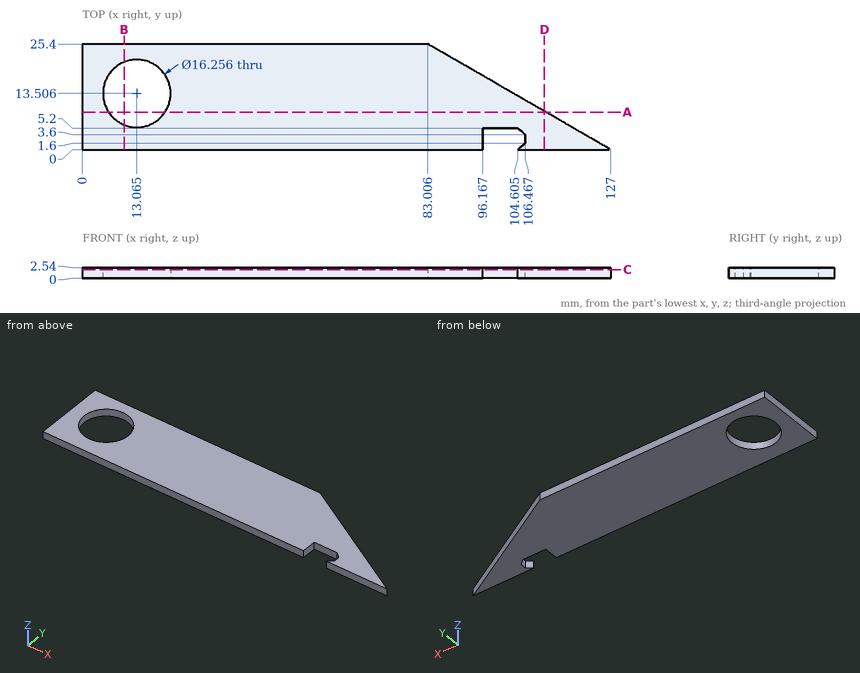
The figure shows three views and two pictorial views of one solid part (mm, origin at its lowest corner). Answer the questions. Give positions to 0.01 mm unless a question says otherwise; leave off trailing zeros. Order: outer loops, then holes, each group sorted by start corner. A loop starts at its lowest first (then second) coordinate and runs counter-clockwise, first axis right, second up. Notation, with made-up numbers: (-39.5, 39) -> (-16.5, 39) arc R28 cw to (-16.5, 59) -> close; hole circle Ø11 at (65.25, -8). An arc over 180 degrees is marked (long way). One line per item, written item: value.
1) Find section C-C, the plane z = 2.05. Determine the outline of the cut face in (x, y) (1 decimal).
Reported:
outline: (0, 0) -> (96.2, 0) -> (96.2, 5.2) -> (104.6, 5.2) -> (106.5, 3.6) -> (106.5, 1.6) -> (104.6, 0) -> (127, 0) -> (83, 25.4) -> (0, 25.4) -> close; hole circle Ø16.3 at (13.1, 13.5)
2) A flat-ended cylindrical pin translates along its axis: P1, Ø12, axis at x = 82, y = 23, coming from the -Z side. Find the tip coordinate at first contact, or state that the pin passes through.
Reported:
P1: stops at z = 0
3) Find section B-B, the plane x = 10. Determine the outline of the cut face in (y, z).
Reported:
outline: (0, 0) -> (5.98, 0) -> (5.98, 2.54) -> (0, 2.54) -> close; (21.03, 0) -> (25.4, 0) -> (25.4, 2.54) -> (21.03, 2.54) -> close
4) Find section D-D, the plane x = 111. Determine the outline of the cut face in (y, z).
Reported:
outline: (0, 0) -> (9.24, 0) -> (9.24, 2.54) -> (0, 2.54) -> close
5) Find section A-A, the plane y = 9. Determine the outline of the cut face in (x, z).
Reported:
outline: (0, 0) -> (6.3, 0) -> (6.3, 2.54) -> (0, 2.54) -> close; (19.83, 0) -> (111.41, 0) -> (111.41, 2.54) -> (19.83, 2.54) -> close
6) Find the intervals of material crossed by line 1 (X direction, y = 3.5, z = 1) (1 decimal); line 2 (X direction, y = 5, z = 0.35) (1 decimal); line 3 (Y direction, x = 11.5, z = 0.65), in increasing order.
Reported:
line 1: x = 0 to 96.2, 106.5 to 120.9
line 2: x = 0 to 96.2, 104.8 to 118.3
line 3: y = 0 to 5.53, 21.48 to 25.4
